Part model, mm, in its own coordinate system. A direction names the side the tool comes from. Round coordinates to 2 decimals unless told otherwise and drop trailing zeros. Write each loop counter-clockwise with the first axis right and the second up, starting at its lowest first coordinate (ties: lowest second). Pieces come first, ordered by that corner, then holes. Notation, with made-up numbers: (85.5, 17) -> (98.5, 17) arc R27 ccw to (98.5, 46) -> close; hole circle Ø11 at (57.5, 65). An arc over 180 degrees is marked (long way). Return JSON: item names as keys, results as strings. Group by question number.
(1) Saw through at C-C (y = 2). List the corners of the cut face in (x, z).
(2) Saw through at A-A (z = 27.65). List the corners of the cut face in (x, y).
(3) Drop flat-ended pins along their axis: pin 1 Ø4 at (x, z) = (31.5, 26.5) entering from -Y; pin 2 Ø4 at (x, z) = (45.5, 5) entering from -Y; pin 3 Ø9 at (x, y) = (39.5, 11) entering from +Z; pin 4 Ø7 at (x, z) = (-15.5, 5.5) entering from +Y. Give the stop position or say it passes through.
(4) Tool access for faces 4 (the flat face through (-35, 8, 40.65)), 5 (the flat face through (-10.06, 4.87, 12.95)), 6 (the cylindrical face through (44.006, 13.262, 27.687)), 7 (the flat face through (43, 8, 37.65)), 8 (the cylindrical face through (29.403, 3.465, 27.764)): list every direction of +Z, -Z, +X, -X, +Y, -Y with a clear straight run to the whole face (end or side of a thin tool).
(5) Mould opens along Y. For faces 1 (the cylindrical face through (-34.597, 3.465, 27.764)), 2 (the flat face through (45, 6, 5)), 3 (the cylindrical face through (-35.994, 13.262, 29.166)) say: +Y half, -Y half, draft (parallel to the pull), parting line (faces both ways), or undercut.
(6) Drill centre lines: L1, parallel to Y at x = 40, z = 29.75; L2, parallel to X at y = 14.75, z = 24; L3, parallel to X at y = 15.5, z = 32. Where is each one in solid material? Low to high. Write a range as from..to.
(7) Saw through at B-B (x = -15.5). List the corners of the cut face in (y, z).
(8) Saw through at D-D (x = 40). List the corners of the cut face in (y, z), plus the area to 3 significant figures.
from build123d import *

# Parameters (mm, degrees)
SKETCH1_R           = 4.2
BOSS_EXTRUDE1_DEPTH = 40.65
SKETCH2_R           = 4.2
BOSS_EXTRUDE2_DEPTH = 18
SKETCH3_R           = 4
CUT_EXTRUDE1_DEPTH  = 22
SKETCH4_R           = 2.6
CUT_EXTRUDE2_DEPTH  = 6
CHAMFER1_SIZE       = 1
CUT_EXTRUDE3_DEPTH  = 22


with BuildPart() as part:
    # Sketch1 → Boss-Extrude1 (new body)
    with BuildSketch(Plane.XY):
        with BuildLine():
            Line((-48.970703673, 12.725586394), (-50, 0))
            Line((-50, 0), (50, 0))
            Line((50, 0), (48.970703673, 12.725586394))
            ThreePointArc((48.970703673, 12.725586394), (43.799691423, 20.158574942), (34.782608696, 19.333404937))
            ThreePointArc((34.782608696, 19.333404937), (0, 8.222771187), (-34.782608696, 19.333404937))
            ThreePointArc((-34.782608696, 19.333404937), (-43.799691423, 20.158574942), (-48.970703673, 12.725586394))
        make_face()
        with Locations((-40, 12)):
            Circle(SKETCH1_R, mode=Mode.SUBTRACT)
        with Locations((40, 12)):
            Circle(SKETCH1_R, mode=Mode.SUBTRACT)
    extrude(amount=BOSS_EXTRUDE1_DEPTH)

    # Sketch2 → Boss-Extrude2 (add)
    with BuildSketch(Plane(origin=(0, 0, 0), x_dir=(-1, 0, 0), z_dir=(0, 0, -1))):
        with Locations((-40, 12)):
            Circle(SKETCH2_R)
        with Locations((40, 12)):
            Circle(SKETCH2_R)
    extrude(amount=-BOSS_EXTRUDE2_DEPTH)

    # Sketch3 → Cut-Extrude1 (cut, through all)
    with BuildSketch(Plane.XZ):
        with Locations((-15.5, 5.5)):
            Circle(SKETCH3_R)
        with Locations((15.5, 5.5)):
            Circle(SKETCH3_R)
        with BuildLine():
            Line((8.764674023, 12.803629506), (32, 37.65))
            Line((32, 37.65), (50, 37.65))
            Line((50, 37.65), (50, 40.65))
            Line((50, 40.65), (-19, 40.65))
            Line((-19, 40.65), (-19, 23.886751346))
            ThreePointArc((-19, 23.886751346), (-17.660254038, 18.886751346), (-14, 15.226497308))
            Line((-14, 15.226497308), (-6, 10.607695155))
            ThreePointArc((-6, 10.607695155), (1.765329298, 9.130559724), (8.764674023, 12.803629506))
        make_face()
    extrude(amount=-CUT_EXTRUDE1_DEPTH, mode=Mode.SUBTRACT)

    # Sketch4 → Cut-Extrude2 (cut)
    with BuildSketch(Plane.XZ):
        with Locations((-32, 27.65)):
            Circle(SKETCH4_R)
        with Locations((-45, 5)):
            Circle(SKETCH4_R)
        with Locations((32, 27.65)):
            Circle(SKETCH4_R)
        with Locations((45, 5)):
            Circle(SKETCH4_R)
    extrude(amount=-CUT_EXTRUDE2_DEPTH, mode=Mode.SUBTRACT)

    # Chamfer1
    chamfer1_edges = [part.edges().sort_by_distance(p)[0] for p in [
        (-34.6, 0, 27.65),
        (-47.6, 0, 5),
        (29.4, 0, 27.65),
        (42.4, 0, 5),
    ]]
    chamfer(chamfer1_edges, length=CHAMFER1_SIZE)

    # Sketch5 → Cut-Extrude3 (cut, through all)
    with BuildSketch(Plane.XZ):
        with BuildLine():
            Line((-50, 5), (-50, 0))
            Line((-50, 0), (-47.331538291, 0))
            Line((-47.331538291, 0), (-48.830222216, 1.786061952))
            ThreePointArc((-48.830222216, 1.786061952), (-49.698463104, 3.289899283), (-50, 5))
        make_face()
        with BuildLine():
            Line((48.830222216, 1.786061952), (47.331538291, 0))
            Line((47.331538291, 0), (50, 0))
            Line((50, 0), (50, 5))
            ThreePointArc((50, 5), (49.698463104, 3.289899283), (48.830222216, 1.786061952))
        make_face()
    extrude(amount=-CUT_EXTRUDE3_DEPTH, mode=Mode.SUBTRACT)


solid = part.part
Computed values:
{
 "1": {"outline": "(-49.84, 3.74) arc R5 ccw to (-48.83, 1.79) -> (-47.33, 0) -> (47.33, 0) -> (48.83, 1.79) arc R5 ccw to (49.84, 3.74) -> (49.84, 37.65) -> (32, 37.65) -> (8.76, 12.8) arc R12 cw to (-6, 10.61) -> (-14, 15.23) arc R10 cw to (-19, 23.89) -> (-19, 40.65) -> (-49.84, 40.65) -> close; hole circle Ø5.2 at (-45, 5); hole circle Ø5.2 at (-32, 27.65); hole circle Ø8 at (-15.5, 5.5); hole circle Ø8 at (15.5, 5.5); hole circle Ø5.2 at (32, 27.65); hole circle Ø5.2 at (45, 5)"},
 "2": {"outline": "(-50, 0) -> (-35.6, 0) -> (-34.6, 1) -> (-34.6, 6) -> (-29.4, 6) -> (-29.4, 1) -> (-28.4, 0) -> (-19, 0) -> (-19, 11.31) arc R60 cw to (-34.78, 19.33) arc R9 ccw to (-48.97, 12.73) -> close; (22.65, 0) -> (28.4, 0) -> (29.4, 1) -> (29.4, 6) -> (34.6, 6) -> (34.6, 1) -> (35.6, 0) -> (50, 0) -> (48.97, 12.73) arc R9 ccw to (34.78, 19.33) arc R60 cw to (22.65, 12.66) -> close; hole circle Ø8.4 at (-40, 12); hole circle Ø8.4 at (40, 12)"},
 "3": {"pin 1": "y = 0.35", "pin 2": "y = 6", "pin 3": "z = 37.65", "pin 4": "through"},
 "4": {"face 4": "+Z, +X, -X, +Y, -Y", "face 5": "+Z, +Y, -Y", "face 6": "+Z", "face 7": "+Z, +X, +Y, -Y", "face 8": "-Y"},
 "5": {"face 1": "draft", "face 2": "-Y half", "face 3": "undercut"},
 "6": {"L1": "0..7.8, 16.2..21", "L2": "-48.57..-43.17, -36.83..-27.22, 27.22..36.83, 43.17..48.57", "L3": "-48.29..-42.32, -37.68..-28.64, 28.64..37.68, 42.32..48.29"},
 "7": {"outline": "(0, 0) -> (10.26, 0) -> (10.26, 1.5) -> (0, 1.5) -> close; (0, 9.5) -> (10.26, 9.5) -> (10.26, 16.29) -> (0, 16.29) -> close"},
 "8": {"outline": "(0, 0) -> (21, 0) -> (21, 37.65) -> (16.2, 37.65) -> (16.2, 18) -> (7.8, 18) -> (7.8, 37.65) -> (0, 37.65) -> close", "area": "626 mm2"}
}
